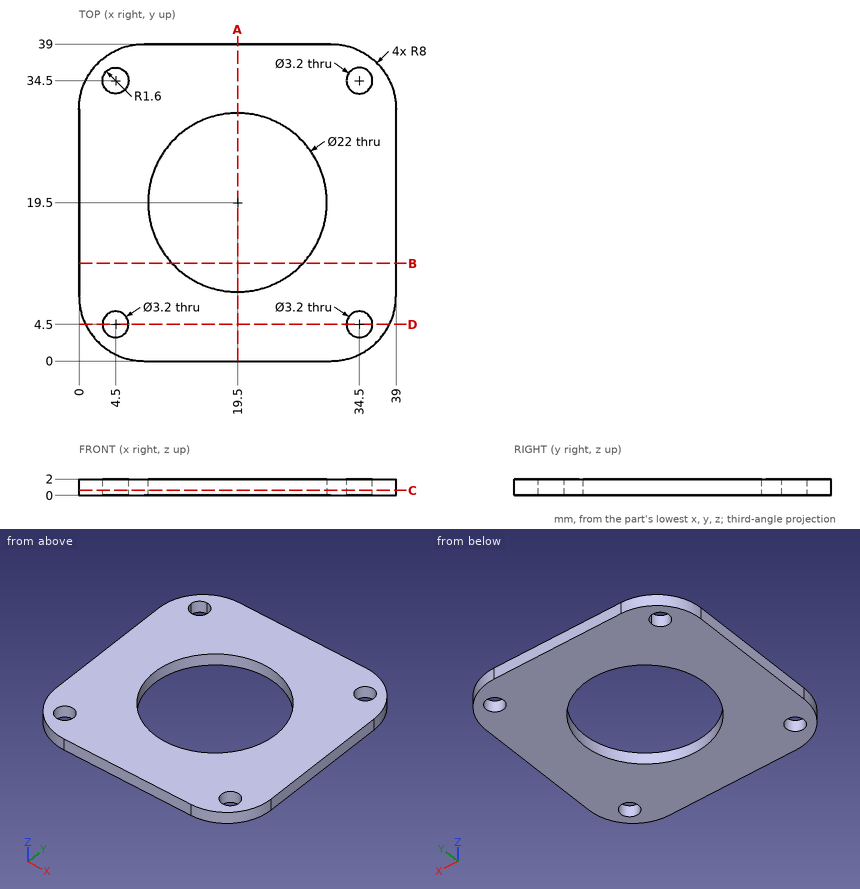
Here's the drawing with two shaded views (mm, measured from the low corner). I have some questions. Give positions to 0.01 mm unless a question says otherwise; leave off trailing zeros. Loops run counter-clockwise (first coordinate to the right, second up) from the corner with the lowest first, then second, coordinate; pieces in that order, holes last. Notation, with made-up numbers: M 63,18.25 L 79,18.25 A26 cw 79,35.25 Z; hole C -38,83.25 d11. An arc over 180 degrees is marked long. Use one line per item in the form item = value. Start each with the question number.
Q1. If we section it at B-B (y = 12): Write out the boundary of the cut face in (x, z), then the cut area to 3 significant figures.
Q2. If we section it at A-A (x = 19.5): Write out the boundary of the cut face in (y, z), then the cut area to 3 significant figures.
Q3. If we section it at D-D (y = 4.5): Write out the boundary of the cut face in (x, z), then the cut area to 3 significant figures.
Q4. Will this pin go through, and if not, where does the flat tip stop? pin 1 Ø1 at (y, z) = (33, 1) entering from -X.
Q5. If we section it at C-C (z = 0.6): Write out the boundary of the cut face in (x, y).
Q6. I need wall thicknesses on line 1 along Y through (x, z) = (19.5, 0.5); line 2 along Y through (x, z) = (5, 1.5); line 3 along X through (y, z) = (17, 1.85). Which ranges of each line are inside material? Lowest first, please.
Taken from the geometry:
q1.outline = M 0,0 L 11.45,0 L 11.45,2 L 0,2 Z; M 27.55,0 L 39,0 L 39,2 L 27.55,2 Z
q1.area = 45.8 mm^2
q2.outline = M 0,0 L 8.5,0 L 8.5,2 L 0,2 Z; M 30.5,0 L 39,0 L 39,2 L 30.5,2 Z
q2.area = 34.0 mm^2
q3.outline = M 0.81,0 L 2.9,0 L 2.9,2 L 0.81,2 Z; M 6.1,0 L 32.9,0 L 32.9,2 L 6.1,2 Z; M 36.1,0 L 38.19,0 L 38.19,2 L 36.1,2 Z
q3.area = 62.0 mm^2
q4.pin_1 = 0.14
q5.outline = M 0,8 A8 ccw 8,0 L 31,0 A8 ccw 39,8 L 39,31 A8 ccw 31,39 L 8,39 A8 ccw 0,31 Z; hole C 4.5,4.5 d3.2; hole C 4.5,34.5 d3.2; hole C 19.5,19.5 d22; hole C 34.5,4.5 d3.2; hole C 34.5,34.5 d3.2
q6.line_1 = 0 to 8.5, 30.5 to 39
q6.line_2 = 0.58 to 2.98, 6.02 to 32.98, 36.02 to 38.42
q6.line_3 = 0 to 8.79, 30.21 to 39
